The listing builds one solid part. Answer for the finished solid, in the listing's coordinates (mm). Face numbers are marked on the shaded views. Give positions to 0.01 mm unless a question says otherwise; leave off trailing zeros. Order: outer loops, then holes, each group sorted by start corner. A loop starts at its lowest first (then second) coordinate and runs counter-clockwise, first axis right, second up. Notation, with made-up numbers: (23.25, 47) - (65.25, 47) arc R22 cw to (65.25, 78) - close; hole circle Ø6 at (3, 27). An arc over 180 degrees is marked (long way). Use a Markdown table: item, result. Add a question column.
1) Flat-ended cylindrical pins translate along their axes: pin 1 (1.5 mm diameter, centred on x = 30, z = 58, fed in from +Y); pin 2 (2.5 mm diameter, centred on x = -30, z = 57, fed in from -Y); pin 3 (6.5 mm diameter, centred on x = 33, y = -1.5, fed in from +Z). Find the tip coordinate at first contact, or state that the pin passes through.
2) Find section A-A, the plane x = 0. Determine the outline of the cut face in (y, z).
3) The mould has two halves that part along Y. Classify the marked faces 1, 2 and 3: released by +Y, released by -Y, zero draft, split by the parting line, or undercut.
4) Find section B-B, the plane z = 57. Determine the outline of the cut face in (x, y), plus the area to 3 significant figures.
5) Find section D-D, the plane y = 7. Determine the outline of the cut face in (x, z) (3 decimals), plus the area to 3 significant figures.
6) Find section C-C, the plane y = 0. Determine the outline of the cut face in (x, z).
7) Straight lines are drawn through the part: line 1 (Y direction, x = 0, z = 58.25); line 2 (X direction, y = -0.5, z = 57.25); line 3 (Y direction, x = 0, z = 63). For each, find the intervals that lie inside material, in ascending order.
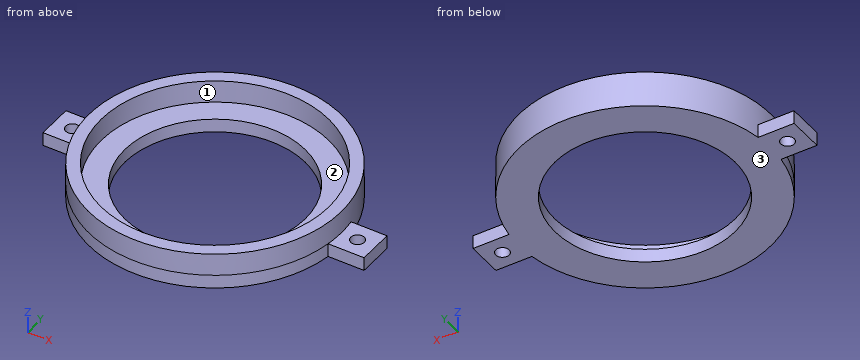
from build123d import *

# Parameters (mm, degrees)
SKETCH023_R     = 20
PAD007_DEPTH    = 3
SKETCH251_R     = 28
SKETCH251_R_2   = 25.25
PAD095_DEPTH    = 5
SKETCH256_R     = 1.5
POCKET125_DEPTH = 8.001


with BuildPart() as part:
    # Sketch023 → Pad007 (new body)
    with BuildSketch(Plane.XY):
        with BuildLine():
            Line((27.712813, -4), (35.712813, -4))
            Line((35.712813, -4), (35.712813, 4))
            Line((35.712813, 4), (27.712813, 4))
            ThreePointArc((27.712813, 4), (0, 28), (-27.712813, 4))
            Line((-35.712813, 4), (-27.712813, 4))
            Line((-35.712813, -4), (-35.712813, 4))
            Line((-27.712813, -4), (-35.712813, -4))
            ThreePointArc((-27.712813, -4), (0, -28), (27.712813, -4))
        make_face()
        Circle(SKETCH023_R, mode=Mode.SUBTRACT)
    extrude(amount=PAD007_DEPTH)

    # Sketch251 → Pad095 (join)
    with BuildSketch(Plane.XY.offset(3)):
        Circle(SKETCH251_R)
        Circle(SKETCH251_R_2, mode=Mode.SUBTRACT)
    extrude(amount=PAD095_DEPTH)

    # Sketch256 (on Face4 of Pad095) → Pocket125 (cut, through all)
    with BuildSketch(Plane(origin=(0, 0, 0), x_dir=(1, 0, 0), z_dir=(0, 0, -1))):
        with Locations((31.712813, 0)):
            Circle(SKETCH256_R)
        with Locations((-31.712813, 0)):
            Circle(SKETCH256_R)
    extrude(amount=-POCKET125_DEPTH, mode=Mode.SUBTRACT)


with BuildPart() as part_1:
    # Body007 placement: moved
    add(part.part.moved(Location((0, 0, 56))))


solid = part_1.part
The answers:
| question | item | result |
|---|---|---|
| 1 | pin 1 | y = 4 |
| 1 | pin 2 | y = -4 |
| 1 | pin 3 | z = 59 |
| 2 | outline | (-28, 56) - (-20, 56) - (-20, 59) - (-25.25, 59) - (-25.25, 64) - (-28, 64) - close; (20, 56) - (28, 56) - (28, 64) - (25.25, 64) - (25.25, 59) - (20, 59) - close |
| 3 | face 1 | undercut |
| 3 | face 2 | undercut |
| 3 | face 3 | zero draft |
| 4 | outline | (-35.71, -4) - (-27.71, -4) arc R28 ccw to (27.71, -4) - (35.71, -4) - (35.71, 4) - (27.71, 4) arc R28 ccw to (-27.71, 4) - (-35.71, 4) - close; hole circle Ø3 at (-31.71, 0); hole circle Ø40 at (0, 0); hole circle Ø3 at (31.71, 0) |
| 4 | area | 1,320 mm2 |
| 5 | outline | (-27.111, 56) - (-18.735, 56) - (-18.735, 59) - (-24.26, 59) - (-24.26, 64) - (-27.111, 64) - close; (18.735, 56) - (27.111, 56) - (27.111, 64) - (24.26, 64) - (24.26, 59) - (18.735, 59) - close |
| 5 | area | 78.8 mm2 |
| 6 | outline | (-35.71, 56) - (-33.21, 56) - (-33.21, 59) - (-35.71, 59) - close; (-30.21, 56) - (-20, 56) - (-20, 59) - (-25.25, 59) - (-25.25, 64) - (-28, 64) - (-28, 59) - (-30.21, 59) - close; (20, 56) - (30.21, 56) - (30.21, 59) - (28, 59) - (28, 64) - (25.25, 64) - (25.25, 59) - (20, 59) - close; (33.21, 56) - (35.71, 56) - (35.71, 59) - (33.21, 59) - close |
| 7 | line 1 | -28 to -20, 20 to 28 |
| 7 | line 2 | -35.71 to -33.13, -30.3 to -19.99, 19.99 to 30.3, 33.13 to 35.71 |
| 7 | line 3 | -28 to -25.25, 25.25 to 28 |
